Source: three-view drawing plus pictorial views. Frame: mm from the lowest corner of the part. Round coordinates to 2 decimals unless told otherwise and drop trailing zeros. Write each loop counter-clockwise with the first axis right and the second up, starting at its lowest first coordinate (ties: lowest second). Pieces come first, ordered by that corner, then holes. Notation, with made-up numbers: (-31.75, 20.25) - (-25.75, 20.25) arc R31 cw to (-25.75, 47.25) - close; hole circle Ø11 at (-3.75, -30.75). An arc over 180 degrees is marked (long way). Write each question's results on one line, items separated by ' | '.
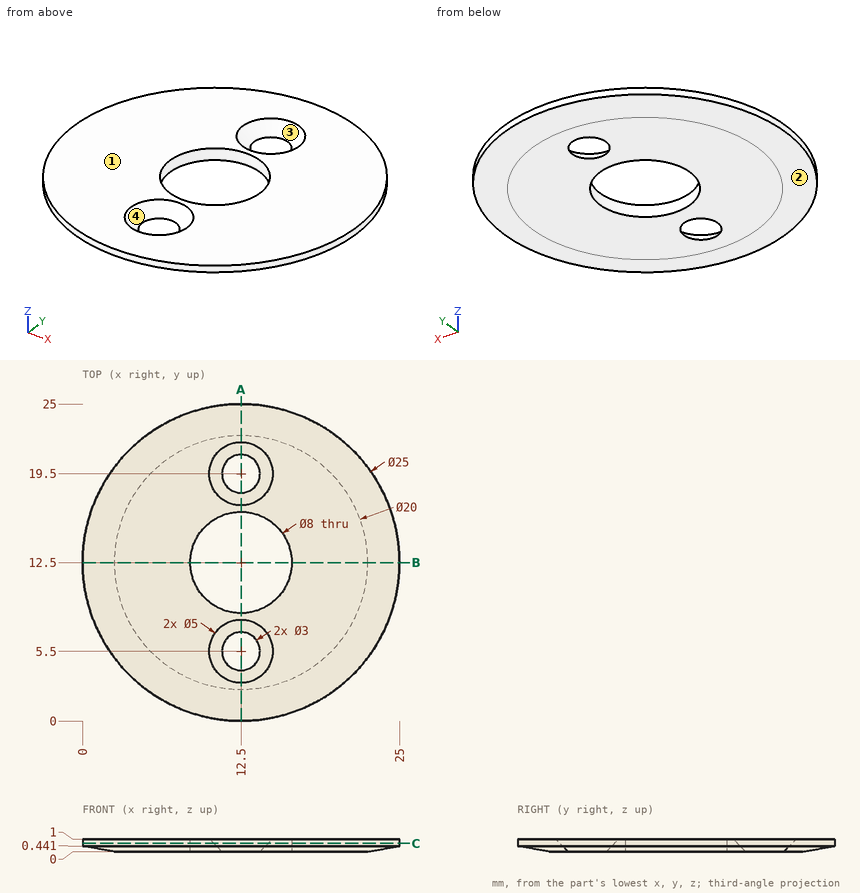
Q1. Section query A-A, the plane x = 12.5. Return loops of the section in (y, z).
Answer block:
outline: (0, 0.44) - (2.5, 0) - (4, 0) - (3, 1) - (0, 1) - close; (7, 0) - (8.5, 0) - (8.5, 1) - (8, 1) - close; (16.5, 0) - (18, 0) - (17, 1) - (16.5, 1) - close; (21, 0) - (22.5, 0) - (25, 0.44) - (25, 1) - (22, 1) - close
Q2. Mould query, pull axis Y, two halves, no side actions, for the marked faces 1, 2, 3 and 4. Classes: pulls with the +Y half, pulls with the -Y half, needs draft (parallel to the pull), parting line crosses it, or undercut.
Answer block:
face 1: needs draft | face 2: parting line crosses it | face 3: undercut | face 4: undercut
Q3. Section query B-B, the plane y = 12.5. Return loops of the section in (x, z).
Answer block:
outline: (0, 0.44) - (2.5, 0) - (8.5, 0) - (8.5, 1) - (0, 1) - close; (16.5, 0) - (22.5, 0) - (25, 0.44) - (25, 1) - (16.5, 1) - close
Q4. Section query C-C, the plane z = 0.65. Return loops of the section in (x, y).
Answer block:
outline: circle Ø25 at (12.5, 12.5); hole circle Ø8 at (12.5, 12.5); hole circle Ø4.3 at (12.5, 5.5); hole circle Ø4.3 at (12.5, 19.5)
Q5. Ray query, line 1 along Y through (x, z) = (12.5, 0.8); line 2 along Y through (x, z) = (12.5, 0.75); line 3 along Y through (x, z) = (9, 0.9) (1 decimal). Return the intervals inside material, ascending.
Answer block:
line 1: 0 to 3.2, 7.8 to 8.5, 16.5 to 17.2, 21.8 to 25 | line 2: 0 to 3.25, 7.75 to 8.5, 16.5 to 17.25, 21.75 to 25 | line 3: 0.5 to 10.6, 14.4 to 24.5
